Work out the finished part from the listing and answer in its coordinate system (mm). A direction names the side the tool comes from. Coordinates: 2 decimals unless noted, no trailing zeros. Order: outer loops, then holes, each group sorted by start corner. A loop starts at its lowest first (then second) coordinate and runs counter-clockwise, first axis right, second up. Notation, with made-up numbers: (52, -9.75) -> (64, -9.75) arc R11 ccw to (64, 8.25) -> close; hole circle Ø8 at (64, 22). An arc over 180 degrees is marked (long way). Use one line per item in the form item = value.
from build123d import *

# Parameters (mm, degrees)
SKETCH_6_W          = 8
SKETCH_6_H          = 6
SKETCH_6_R          = 1.5
EXTRUDE_1_DEPTH     = 1.5
SKETCH_7_W          = 8
SKETCH_7_H          = 25
EXTRUDE_2_DEPTH     = 2
SKETCH_8_W          = 35
SKETCH_8_H          = 2
EXTRUDE_3_DEPTH     = 22
SKETCH_9_W          = 22
SKETCH_9_H          = 12
CUT_EXTRUDE_1_DEPTH = 10
SKETCH_14_W         = 8
SKETCH_14_H         = 6
CUT_EXTRUDE_2_DEPTH = 4.6
RIB_3_REACH         = 76.814
SKETCH_15_WALL_W    = 159.949062396
SKETCH_15_WALL_H    = 2
FILLET_2_R          = 3
SKETCH_16_W         = 8
SKETCH_16_H         = 2
EXTRUDE_4_DEPTH     = 1.8
SKETCH_17_R         = 1
CUT_EXTRUDE_3_DEPTH = 10


with BuildPart() as part:
    # 草图6 → 凸台-拉伸1 (new body)
    with BuildSketch(Plane(origin=(0, 0, 0), x_dir=(1, 0, 0), z_dir=(0, 1, 0))):
        with Locations((1, 0)):
            Rectangle(SKETCH_6_W, SKETCH_6_H)
        with Locations(Location((0, 0, 0), (0, 0, 270))):
            Circle(SKETCH_6_R, mode=Mode.SUBTRACT)
    extrude(amount=EXTRUDE_1_DEPTH)

    # 草图7 → 凸台-拉伸2 (add)
    with BuildSketch(Plane(origin=(0, 0, -3), x_dir=(-1, 0, 0), z_dir=(0, 0, -1))):
        with Locations((-1, 12.5)):
            Rectangle(SKETCH_7_W, SKETCH_7_H)
    extrude(amount=EXTRUDE_2_DEPTH)

    # 镜向1: part across plane


with BuildPart() as part_1:
    add(part.part)
    add(part.part.mirror(Plane(origin=(-3, 25, -5), x_dir=(0, 0, 1), z_dir=(0, -1, 0))))

    # 草图8 → 凸台-拉伸3 (add)
    with BuildSketch(Plane(origin=(0, 50, 0), x_dir=(1, 0, 0), z_dir=(0, 1, 0))):
        with Locations((2.8, 4)):
            Rectangle(SKETCH_8_W, SKETCH_8_H)
    extrude(amount=EXTRUDE_3_DEPTH)

    # 草图9 → 切除-拉伸1 (cut)
    with BuildSketch(Plane(origin=(0, 0, -5), x_dir=(-1, 0, 0), z_dir=(0, 0, -1))):
        with Locations((-1.3, 64.5)):
            Rectangle(SKETCH_9_W, SKETCH_9_H)
    extrude(amount=-CUT_EXTRUDE_1_DEPTH, mode=Mode.SUBTRACT)

    # 草图14 → 切除-拉伸2 (cut)
    with BuildSketch(Plane(origin=(0, 50, 0), x_dir=(1, 0, 0), z_dir=(0, 1, 0))):
        with Locations((1, 0)):
            Rectangle(SKETCH_14_W, SKETCH_14_H)
    extrude(amount=-CUT_EXTRUDE_2_DEPTH, mode=Mode.SUBTRACT)

    # 草图15 wall → 筋3 (add, up to next)
    with BuildSketch(Plane(origin=(5, 5, -0.75), x_dir=(0, 0.841178475377, -0.540757591313), z_dir=(0, 0.540757591313, 0.841178475377)), mode=Mode.PRIVATE) as rib_3_sk1:
        with Locations((0, 1)):
            Rectangle(SKETCH_15_WALL_W, SKETCH_15_WALL_H)
    rib_3_tool1 = extrude(rib_3_sk1.sketch, amount=-RIB_3_REACH, mode=Mode.PRIVATE) - part_1.part
    add(rib_3_tool1.solids().sort_by_distance((5, 5, -0.75))[0])

    # 圆角2
    fillet_2_edges = [part_1.edges().sort_by_distance(p)[0] for p in [
        (-3, 50, -4),
        (5, 50, -4),
        (-14.7, 50, -4),
        (20.3, 50, -4),
        (-14.7, 72, -4),
        (20.3, 72, -4),
    ]]
    fillet(fillet_2_edges, radius=FILLET_2_R)

    # 草图16 → 凸台-拉伸4 (add)
    with BuildSketch(Plane(origin=(0, 0, 0), x_dir=(-1, 0, 0), z_dir=(0, -1, 0))):
        with Locations((-1, 4)):
            Rectangle(SKETCH_16_W, SKETCH_16_H)
    extrude(amount=EXTRUDE_4_DEPTH)

    # 草图17 → 切除-拉伸3 (cut)
    with BuildSketch(Plane(origin=(0, 0, -5), x_dir=(-1, 0, 0), z_dir=(0, 0, -1))):
        with Locations((-15.7, 64.5)):
            Circle(SKETCH_17_R)
        with Locations((12.1, 64.5)):
            Circle(SKETCH_17_R)
    extrude(amount=-CUT_EXTRUDE_3_DEPTH, mode=Mode.SUBTRACT)


solid = part_1.part
(1) Each of these flat-tipped pins is pushed along its axis until it touches: P1, Ø1.8, axis at x = 2, z = -1, coming from the -Y side; P2, Ø1.3, axis at y = 4.5, z = 0, coming from the -X side; P3, Ø0.9, axis at x = 1, y = -1, coming from the +Z side; P4, Ø1.8, axis at x = -12.1, y = 64.5, coming from the -Z side. Where does it stop, or does it pass through?
Data:
P1 = 0
P2 = 3
P3 = -3
P4 = through
(2) Straight lines are drawn through the part: line 1 along X through (y, z) = (64.5, -3.7); line 2 along Y through (x, z) = (15.7, -4.3); line 3 along Y through (x, z) = (-2, 0). For each, find the intervals that lie inside material, in ascending order.
Data:
line_1 = -14.7 to -13.1, -11.1 to -9.7, 12.3 to 14.7, 16.7 to 20.3
line_2 = 50 to 63.5, 65.5 to 72
line_3 = 0 to 1.5
(3) Section A-A on x = 0 is taken. Write down the section's boundary in (y, z), plus the area to 3 significant figures.
Data:
outline = (-1.8, -5) -> (58.5, -5) -> (58.5, -3) -> (1.5, -3) -> (1.5, -1.5) -> (0, -1.5) -> (0, -3) -> (-1.8, -3) -> close; (0, 1.5) -> (1.5, 1.5) -> (1.5, 3) -> (0, 3) -> close; (70.5, -5) -> (72, -5) -> (72, -3) -> (70.5, -3) -> close
area = 128 mm²
(4) Which of the six approach directions +Z, -Z, +X, -X, +Y, -Y give full straight-line access (tool end or side, diameter ignored) to faces 4 (the flat face through (1, -1.8, -4)), 5 (the flat face through (5, 19, -4)), 6 (the flat face through (1, -1, -3)), 7 (the flat face through (1, 70.5, -4))?
Data:
face_4 = +Z, -Z, +X, -X, -Y
face_5 = +Z, -Z, +X, -Y
face_6 = +Z, +X, -X, -Y
face_7 = +Z, -Z
(5) Section D-D on z = 0.25 is taken. Write down the section's boundary in (x, y), plus the area to 3 significant figures.
Data:
outline = (-3, 0) -> (-1.48, 0) -> (-1.48, 1.5) -> (-3, 1.5) -> close; (1.48, 0) -> (5, 0) -> (5, 3.44) -> (3, 3.44) -> (3, 1.5) -> (1.48, 1.5) -> close
area = 11.5 mm²
(6) Section B-B on y = 61.5 is taken. Write down the section's boundary in (x, z).
Data:
outline = (-14.7, -5) -> (-9.7, -5) -> (-9.7, -3) -> (-14.7, -3) -> close; (12.3, -5) -> (20.3, -5) -> (20.3, -3) -> (12.3, -3) -> close
(7) Section C-C on x = 15.7 is taken. Write down the section's boundary in (y, z).
Data:
outline = (50, -5) -> (63.5, -5) -> (63.5, -3) -> (50, -3) -> close; (65.5, -5) -> (72, -5) -> (72, -3) -> (65.5, -3) -> close
(8) The mould has two halves that part along Y. Classify faces 1 (the flat face through (1, 1, 3)), 2 (the cylindrical face through (15.83, 65.49, -4.01)), 3 (the flat face through (13, 50, -4)): released by +Y, released by -Y, zero draft, split by the parting line, or undercut.
Data:
face_1 = zero draft
face_2 = undercut
face_3 = released by -Y
